Geometry: see drawing. Coordinates: mm, zero at the bounding-box minimum. A direction names the side the tool comes from. Round coordinates to 2 decimals unless told otherwise and drop trailing zeros. Write each loop counter-clockwise with the first axis right and the second up, starting at its lowest first coordinate (ties: lowest second). Pieces come first, ordered by that corner, then holes. Notation, with made-up numbers: (46.25, 43.25) - (71.25, 43.25) arc R6 cw to (71.25, 48.25) - close; hole circle Ø9 at (1, 81.5). An arc over 180 degrees is marked (long way). One line per item, written item: value. Start each with the question number.
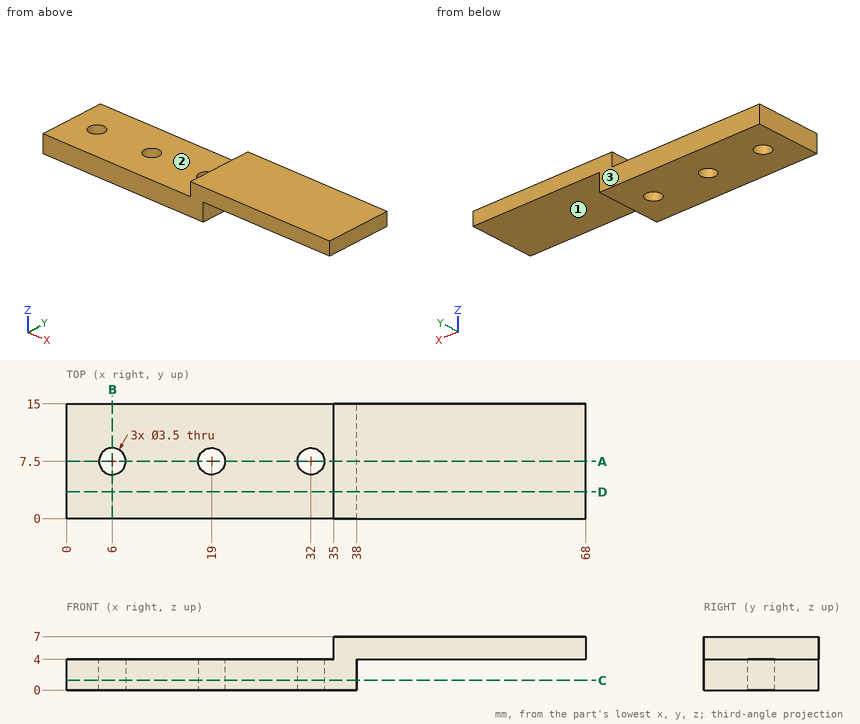
Q1. Cut plane A-A, the plane y = 7.5. Output: boundary loops of the cut face in (x, z), and give its area (3 significant figures).
Q2. Cut plane C-C, the plane z = 1.25. Output: boundary loops of the cut face in (x, y).
Q3. Material intervals for probe 1 along Y at (x, z) = (32, 2.25); probe 2 along Z at (x, y) = (9.5, 4.5); probe 3 along X at (y, z) = (8, 0.75), sorted ascending. Write a range as from..to.
Q4. Access query for the marked faces 1, 2 and 3. Directions: +Z, -Z, +X, -X, +Y, -Y. A direction counts if a zero-diameter tool reaches every point of the face in a straight line with its end or side. Return the directions, or none.
Q5. Cut plane B-B, the plane x = 6. Output: boundary loops of the cut face in (y, z).
Q6. Contact query for flat-ended pins moving along their axis: pin 1 Ø1.5 at (y, z) = (6, 1) entering from -X; pin 2 Ø4.5 at (x, y) = (32, 7.5) entering from +Z; pin 3 Ø1.5 at (y, z) = (5, 5.5) entering from -X. Output: stop coordinate, or through.
Q7. Cut plane D-D, the plane y = 3.5. Output: boundary loops of the cut face in (x, z).
A:
1. outline: (0, 0) - (4.25, 0) - (4.25, 4) - (0, 4) - close; (7.75, 0) - (17.25, 0) - (17.25, 4) - (7.75, 4) - close; (20.75, 0) - (30.25, 0) - (30.25, 4) - (20.75, 4) - close; (33.75, 0) - (38, 0) - (38, 4) - (68, 4) - (68, 7) - (35, 7) - (35, 4) - (33.75, 4) - close
1. area: 209 mm²
2. outline: (0, 0) - (38, 0) - (38, 15) - (0, 15) - close; hole circle Ø3.5 at (6, 7.5); hole circle Ø3.5 at (19, 7.5); hole circle Ø3.5 at (32, 7.5)
3. probe 1: y = 0..5.75, 9.25..15
3. probe 2: z = 0..4
3. probe 3: x = 0..4.32, 7.68..17.32, 20.68..30.32, 33.68..38
4. face 1: -Z, +X, +Y, -Y
4. face 2: +Z, -X, +Y, -Y
4. face 3: +Z, -Z, +X, -X, +Y
5. outline: (0, 0) - (5.75, 0) - (5.75, 4) - (0, 4) - close; (9.25, 0) - (15, 0) - (15, 4) - (9.25, 4) - close
6. pin 1: stops at x = 0
6. pin 2: stops at z = 4
6. pin 3: stops at x = 35
7. outline: (0, 0) - (38, 0) - (38, 4) - (68, 4) - (68, 7) - (35, 7) - (35, 4) - (0, 4) - close
